Geometry: final body of the model. Coordinates: model frame, mm. Face numbers are marked on the shaded views. A direction names the side the tool comes from. Give positions to 0.01 mm unless a question says otherwise; leave off trailing zeros. Order: outer loops, then holes, each group sorted by start corner. A loop starts at its lowest first (then second) coordinate and runs counter-clockwise, first axis right, second up. Notation, with made-up numbers: (17, 60.5) -> (47, 60.5) arc R24 ccw to (47, 91.5) -> close; hole circle Ø8 at (-21.75, -38.5). An arc over 180 degrees is marked (long way). Write item = value, one per line.
```python
from build123d import *

# Parameters (mm, degrees)
EXTRUDE_1_DEPTH     = 24
SKETCH_2_R          = 1.6
CUT_EXTRUDE_1_DEPTH = 24
SKETCH_3_R          = 1.6
CUT_EXTRUDE_2_DEPTH = 24
FILLET_1_R          = 2
SKETCH_4_R          = 1.6
CUT_EXTRUDE_3_DEPTH = 4
SKETCH_5_R          = 1.6
CUT_EXTRUDE_4_DEPTH = 4


with BuildPart() as part:
    # 草图1 → 凸台-拉伸1 (new body)
    with BuildSketch(Plane.XY):
        Polygon((6, 129.691622655), (3, 129.691622655), (3, 101.691622655), (26, 101.691622655), (26, 104.691622655), (6, 104.691622655), align=None)
    extrude(amount=-EXTRUDE_1_DEPTH)

    # 草图2 → 切除-拉伸1 (cut)
    with BuildSketch(Plane(origin=(6, 0, 0), x_dir=(0, 0, -1), z_dir=(1, 0, 0))):
        with Locations(Location((6, 125.691622655, 0), (0, 0, 90))):
            Circle(SKETCH_2_R)
        with Locations(Location((18, 125.691622655, 0), (0, 0, 90))):
            Circle(SKETCH_2_R)
    extrude(amount=-CUT_EXTRUDE_1_DEPTH, mode=Mode.SUBTRACT)

    # 草图3 → 切除-拉伸2 (cut)
    with BuildSketch(Plane(origin=(0, 104.691622655, 0), x_dir=(1, 0, 0), z_dir=(0, 1, 0))):
        with Locations(Location((22, 6, 0), (0, 0, 180))):
            Circle(SKETCH_3_R)
        with Locations(Location((22, 18, 0), (0, 0, 180))):
            Circle(SKETCH_3_R)
    extrude(amount=-CUT_EXTRUDE_2_DEPTH, mode=Mode.SUBTRACT)

    # 圆角1
    fillet_1_edges = [part.edges().sort_by_distance(p)[0] for p in [
        (4.5, 129.691622655, -24),
        (4.5, 129.691622655, 0),
        (26, 103.191622655, -24),
        (26, 103.191622655, 0),
    ]]
    fillet(fillet_1_edges, radius=FILLET_1_R)

    # 草图4 → 切除-拉伸3 (cut)
    with BuildSketch(Plane.ZY.offset(-3)):
        with Locations(Location((-18, 112.691622655, 0), (0, 0, 270))):
            Circle(SKETCH_4_R)
        with Locations(Location((-6, 112.691622655, 0), (0, 0, 270))):
            Circle(SKETCH_4_R)
    extrude(amount=-CUT_EXTRUDE_3_DEPTH, mode=Mode.SUBTRACT)

    # 草图5 → 切除-拉伸4 (cut)
    with BuildSketch(Plane(origin=(0, 104.691622655, 0), x_dir=(1, 0, 0), z_dir=(0, 1, 0))):
        with Locations(Location((12, 18, 0), (0, 0, 180))):
            Circle(SKETCH_5_R)
        with Locations(Location((12, 6, 0), (0, 0, 180))):
            Circle(SKETCH_5_R)
    extrude(amount=-CUT_EXTRUDE_4_DEPTH, mode=Mode.SUBTRACT)


solid = part.part
```
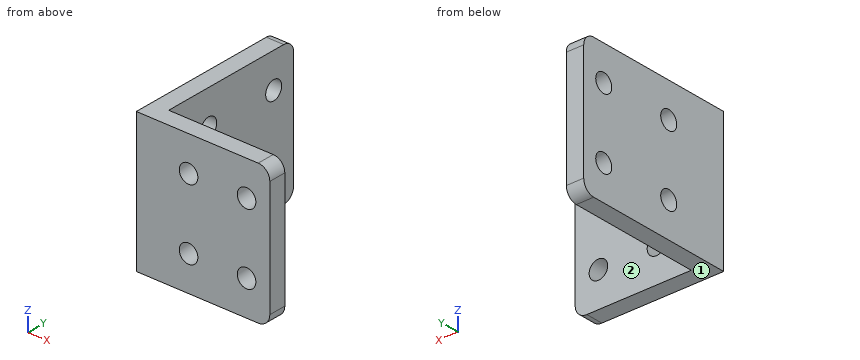
1) Section query C-C (y = 112.75). Output: boundary loops of the cut face in (x, z), plus the area to 3 significant figures.
Check sheet entries:
outline = (3, -24) -> (6, -24) -> (6, -19.6) -> (3, -19.6) -> close; (3, -16.4) -> (6, -16.4) -> (6, -7.6) -> (3, -7.6) -> close; (3, -4.4) -> (6, -4.4) -> (6, 0) -> (3, 0) -> close
area = 52.8 mm²
2) Section query A-A (x = 22). Output: boundary loops of the cut face in (y, z).
Check sheet entries:
outline = (101.69, -24) -> (104.69, -24) -> (104.69, -19.6) -> (101.69, -19.6) -> close; (101.69, -16.4) -> (104.69, -16.4) -> (104.69, -7.6) -> (101.69, -7.6) -> close; (101.69, -4.4) -> (104.69, -4.4) -> (104.69, 0) -> (101.69, 0) -> close
3) Line query: line 1 (Z direction, x = 22, y = 103); line 2 (Y direction, x = 8.25, z = -11); line 3 (X direction, y = 120.75, z = -1.25). Output: solid intervals per line, ascending. Write a range as from..to.
Check sheet entries:
line_1 = -24..-19.6, -16.4..-7.6, -4.4..0
line_2 = 101.69..104.69
line_3 = 3..6
4) Section query D-D (z = -6.5). Output: boundary loops of the cut face in (x, y).
Check sheet entries:
outline = (3, 101.69) -> (10.48, 101.69) -> (10.48, 104.69) -> (6, 104.69) -> (6, 111.17) -> (3, 111.17) -> close; (3, 114.21) -> (6, 114.21) -> (6, 124.17) -> (3, 124.17) -> close; (3, 127.21) -> (6, 127.21) -> (6, 129.69) -> (3, 129.69) -> close; (13.52, 101.69) -> (20.48, 101.69) -> (20.48, 104.69) -> (13.52, 104.69) -> close; (23.52, 101.69) -> (26, 101.69) -> (26, 104.69) -> (23.52, 104.69) -> close
5) Reachability of the marked faces 1 and 2 from +Z, -Z, +X, -X, +Y, -Y: full face, straight path, thin tool, end or side. Return the list, or none.
Check sheet entries:
face_1 = -Z, +X, -X, +Y, -Y
face_2 = +Z, -Z, +X, +Y
6) Section query B-B (z = -18). Output: boundary loops of the cut face in (x, y).
Check sheet entries:
outline = (3, 101.69) -> (10.4, 101.69) -> (10.4, 104.69) -> (6, 104.69) -> (6, 111.09) -> (3, 111.09) -> close; (3, 114.29) -> (6, 114.29) -> (6, 124.09) -> (3, 124.09) -> close; (3, 127.29) -> (6, 127.29) -> (6, 129.69) -> (3, 129.69) -> close; (13.6, 101.69) -> (20.4, 101.69) -> (20.4, 104.69) -> (13.6, 104.69) -> close; (23.6, 101.69) -> (26, 101.69) -> (26, 104.69) -> (23.6, 104.69) -> close
7) First-contact query: P1, Ø12, axis at x = 14.5, y = 106.5, coming from the -Z side; P2, Ø1, axis at x = 15, z = -10.5, coming from the +Y side; P3, Ø1, axis at y = 117, z = -7, coming from the +X side. Flat tips, straight axial feed; report the tip coordinate or a pass-through.
Check sheet entries:
P1 = -24
P2 = 104.69
P3 = 6
